Model file for the job. Use its own axes, mm. Coordinates: 2 decimals unless noted, no trailing zeros. Write each loop counter-clockwise with the first axis right and the second up, starting at its lowest first coordinate (ties: lowest second). Pieces come first, ordered by that corner, then holes. Notation, with made-up numbers: M -35.5,18 L -19.5,18 A22 cw -19.5,40 Z; hole C -33.5,38.25 d9. An arc over 180 degrees is marked long. Answer in a Markdown table with one row per item. Add a question column.
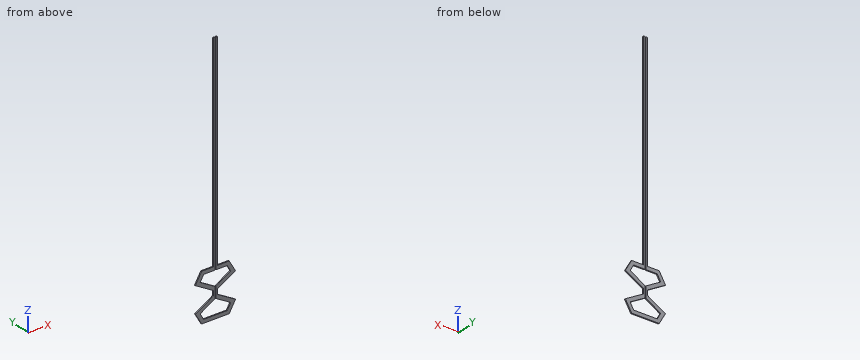
```python
from build123d import *

# Parameters (mm, degrees)
EXTRUDE_1_DEPTH          = 1
EXTRUDE_1_2_DEPTH        = 1
CUT_EXTRUDE_1_DEPTH      = 2
CUT_EXTRUDE_1_DEPTH_BACK = 2
SKETCH_2_W               = 1.200484238
SKETCH_2_H               = 35
SKETCH_3_W               = 1
SKETCH_3_H               = 179.349364905
EXTRUDE_2_DEPTH          = 1


with BuildPart() as part:
    # Sketch 1 → Extrude 1 (new body)
    with BuildSketch(Plane(origin=(0, 0, 0), x_dir=(1, 0, 0), z_dir=(0, 1, 0))):
        Polygon((11.922649731, 20.650635095), (-11.922649731, 20.650635095), (-17.383974596, 11.191342951), (0, 1.154700538), (17.383974596, 11.191342951), align=None)
        Polygon((10.190598923, 17.650635095), (-10.190598923, 17.650635095), (-13.285898385, 12.289419162), (0, 4.618802154), (13.285898385, 12.289419162), align=None, mode=Mode.SUBTRACT)
    extrude(amount=EXTRUDE_1_DEPTH)


with BuildPart() as body_2:
    # Sketch 1 → Extrude 1 2 (new body)
    with BuildSketch(Plane(origin=(0, 0, 0), x_dir=(1, 0, 0), z_dir=(0, 1, 0))):
        Polygon((0, -1.154700538), (-17.383974596, -11.191342951), (-11.922649731, -20.650635095), (11.922649731, -20.650635095), (17.383974596, -11.191342951), align=None)
        Polygon((0, -4.618802154), (-13.285898385, -12.289419162), (-10.190598923, -17.650635095), (10.190598923, -17.650635095), (13.285898385, -12.289419162), align=None, mode=Mode.SUBTRACT)
    extrude(amount=EXTRUDE_1_2_DEPTH)


with BuildPart() as cut_extrude_1_tool:
    # Sketch 2 → Cut-Extrude 1 (new, two sides: drawn at the far end of the back side and taken through both)
    with BuildSketch(Plane(origin=(0, 0, 0), x_dir=(1, 0, 0), z_dir=(0, 1, 0)).offset(-CUT_EXTRUDE_1_DEPTH_BACK)):
        with Locations((0, -4.618802154)):
            Rectangle(SKETCH_2_W, SKETCH_2_H)
    extrude(amount=CUT_EXTRUDE_1_DEPTH + CUT_EXTRUDE_1_DEPTH_BACK)


with BuildPart() as part_1:
    add(part.part)

    # Cut-Extrude 1: cut by cut_extrude_1_tool
    add(cut_extrude_1_tool.part, mode=Mode.SUBTRACT)



with BuildPart() as body_2_1:
    add(body_2.part)

    # Cut-Extrude 1: cut by cut_extrude_1_tool
    add(cut_extrude_1_tool.part, mode=Mode.SUBTRACT)


with BuildPart() as part_2:
    add(part_1.part)

    add(body_2_1.part)  # Extrude 2 merges body 2
    # Sketch 3 → Extrude 2 (add)
    with BuildSketch(Plane(origin=(0, 0, 0), x_dir=(1, 0, 0), z_dir=(0, 1, 0))):
        with Locations((-1.100242119, -110.325317548)):
            Rectangle(SKETCH_3_W, SKETCH_3_H)
        with Locations((1.100242119, -110.325317548)):
            Rectangle(SKETCH_3_W, SKETCH_3_H)
        Polygon((-0.600242119, -1.501250487), (-0.600242119, 1.501250487), (-1.600242119, 2.078600756), (-1.600242119, -2.078600756), align=None)
        Polygon((0.600242119, -1.501250487), (0.600242119, 1.501250487), (1.600242119, 2.078600756), (1.600242119, -2.078600756), align=None)
    extrude(amount=EXTRUDE_2_DEPTH)


solid = part_2.part
```
1) Drill centre lines: probe 1 along X at (y, z) = (0.3, 131); probe 2 along Z at (x, y) = (5, 0.15); probe 3 along Z at (x, y) = (7, 0.1). Where is each one in solid material? Low to high.
2) Slice it at A-A (z = 171). Give the cut face in (x, y).
3) Slice it at C-C (x = -8). Give the cut face in (y, z).
Ans:
| question | item | result |
|---|---|---|
| 1 | probe 1 | x = -1.6 to -0.6, 0.6 to 1.6 |
| 1 | probe 2 | z = -20.65 to -17.65, -7.51 to -4.04, 4.04 to 7.51, 17.65 to 20.65 |
| 1 | probe 3 | z = -20.65 to -17.65, -8.66 to -5.2, 5.2 to 8.66, 17.65 to 20.65 |
| 2 | outline | M -1.6,0 L -0.6,0 L -0.6,1 L -1.6,1 Z; M 0.6,0 L 1.6,0 L 1.6,1 L 0.6,1 Z |
| 3 | outline | M 0,-20.65 L 1,-20.65 L 1,-17.65 L 0,-17.65 Z; M 0,-9.24 L 1,-9.24 L 1,-5.77 L 0,-5.77 Z; M 0,5.77 L 1,5.77 L 1,9.24 L 0,9.24 Z; M 0,17.65 L 1,17.65 L 1,20.65 L 0,20.65 Z |
